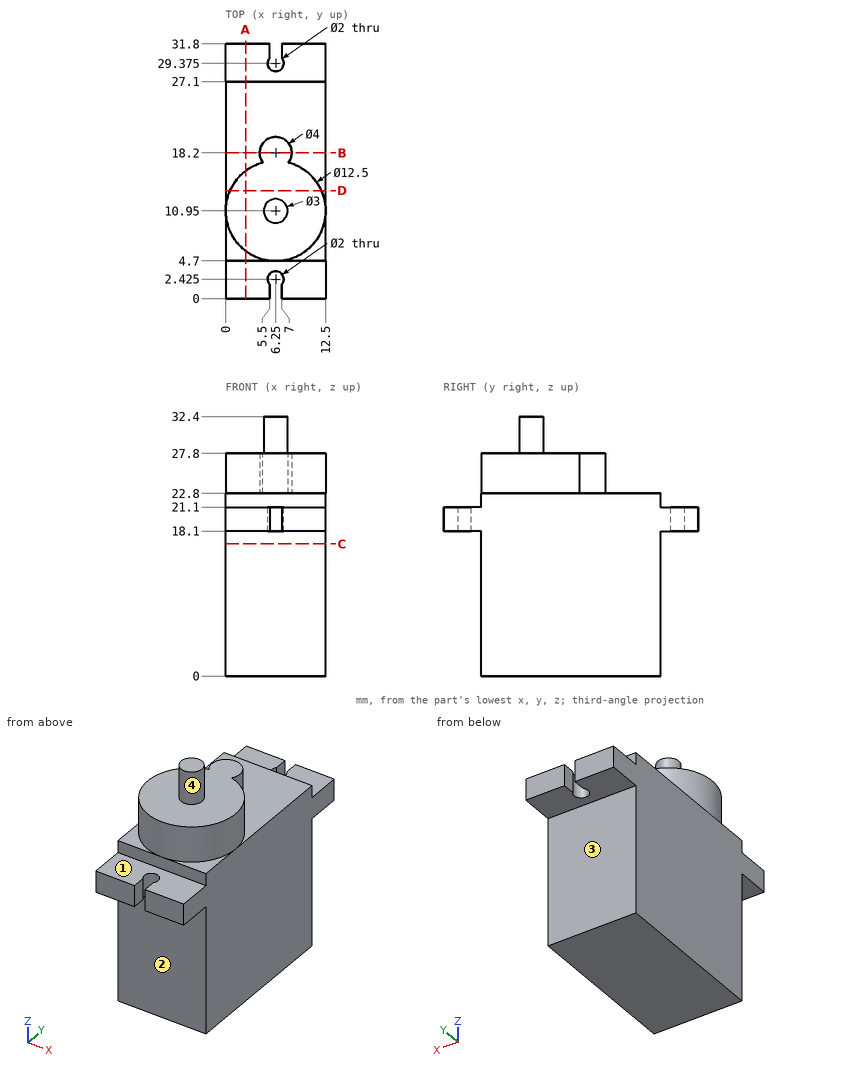
Input: dimensioned drawing with shaded views. Units: mm. Origin: part minimum x, y, z. A direction names the side the tool comes from. Give positions to 0.01 mm unless a question says otherwise; leave off trailing zeros. Loops run counter-clockwise (first coordinate to the right, second up) from the corner with the lowest first, then second, coordinate; pieces in that order, holes last. Notation, with made-up numbers: (64, -15.5) -> (120, -15.5) arc R25 ccw to (120, 22.5) -> close; hole circle Ø9 at (39.5, 81.25). An arc over 180 degrees is marked (long way). Use a Markdown table: item, result.
Q1. First-contact query: P1, Ø5, axis at x = 6.5, y = 1.5, coming from the -Z side; P2, Ø4, axis at x = 3, y = 15.5, coming from the +Z side; P3, Ø1.5, axis at x = 2.5, z = 27, coming from the +Y side; P4, Ø1.8, axis at x = 6.25, y = 2.425, coming from the -Z side. Flat tips, straight axial feed; report the tip coordinate or a pass-through.
Entries:
| item | result |
|---|---|
| P1 | stops at z = 18.1 |
| P2 | stops at z = 27.8 |
| P3 | stops at y = 16.43 |
| P4 | passes through |
Q2. Section query D-D, the plane y = 13.5. Return the cut outline in (x, z).
Entries:
| item | result |
|---|---|
| outline | (0, 0) -> (12.5, 0) -> (12.5, 22.8) -> (11.96, 22.8) -> (11.96, 27.8) -> (0.54, 27.8) -> (0.54, 22.8) -> (0, 22.8) -> close |
Q3. Section query A-A, the plane x = 2.5. Return the cut outline in (y, z).
Entries:
| item | result |
|---|---|
| outline | (0, 18.1) -> (4.7, 18.1) -> (4.7, 0) -> (27.1, 0) -> (27.1, 18.1) -> (31.8, 18.1) -> (31.8, 21.1) -> (27.1, 21.1) -> (27.1, 22.8) -> (15.95, 22.8) -> (15.95, 27.8) -> (5.95, 27.8) -> (5.95, 22.8) -> (4.7, 22.8) -> (4.7, 21.1) -> (0, 21.1) -> close |
Q4. Section query C-C, the plane z = 16.5. Return the cut outline in (x, y).
Entries:
| item | result |
|---|---|
| outline | (0, 4.7) -> (12.5, 4.7) -> (12.5, 27.1) -> (0, 27.1) -> close |
Q5. Access query for the marked faces 1, 2, 3 and 4. Directions: +Z, -Z, +X, -X, +Y, -Y. A direction counts if a zero-diameter tool reaches every point of the face in a straight line with its end or side. Return the directions, or none.
Entries:
| item | result |
|---|---|
| face 1 | +Z, +X, -X, -Y |
| face 2 | -Z, +X, -X, -Y |
| face 3 | -Z, +X, -X, +Y |
| face 4 | +Z |
Q6. Ray query, probe 1 along Y at (x, z) = (3, 14.5); probe 2 along Z at (x, y) = (6.25, 20); probe 3 along Z at (x, y) = (11.25, 2.5). Return the intervals inside material, ascending. Write a range as from..to.
Entries:
| item | result |
|---|---|
| probe 1 | y = 4.7..27.1 |
| probe 2 | z = 0..27.8 |
| probe 3 | z = 18.1..21.1 |
Q7. Section query B-B, the plane y = 18.2. Return the cut outline in (x, z).
Entries:
| item | result |
|---|---|
| outline | (0, 0) -> (12.5, 0) -> (12.5, 22.8) -> (8.25, 22.8) -> (8.25, 27.8) -> (4.25, 27.8) -> (4.25, 22.8) -> (0, 22.8) -> close |
